Check sheet for the drawn part. Datum: minimum x, y, z corner. Units: mm. A direction names the side the tool comes from. Give positions to 0.01 mm unless a question says otherwise; leave off trailing zeros. Write each loop counter-clockwise with the first axis right and the second up, starting at its lowest first coordinate (ties: lowest second). Pieces come first, ordered by that corner, then holes. Notation, with made-up numbers: (79.25, -36.75) - (121.25, -36.75) arc R28 cw to (121.25, -8.75) - close; hole circle Ø11 at (-3.75, 48.5). An arc over 180 degrees is marked (long way). One line per question, with ' | ' between items. Start each with the question number.
Q1. Section check A-A on x = 37.5. Record the boundary of the cut face in (y, z).
Q2. Thickness scan on L1, parallel to Y at x = 2.5, z = 0.45; L2, parallel to Y at x = 19.5, z = 2.2; L3, parallel to Z at x = 13, y = 2. Record the ranges inside material, lowest first. Write a range as [from, to].
Q3. Section check D-D on y = 24. Record the boundary of the cut face in (x, z), and give its area (3 significant figures).
Q4. Set-up check for the marked faces 1, 2, 3, 4 and 5: record each of +Z, -Z, +X, -X, +Y, -Y from which the full face is reachable in a straight line by a thin tool's end or side.
Q5. Section check B-B on y = 2.5. Record the boundary of the cut face in (x, z), and give its area (3 significant figures).
Q6. Section check C-C on x = 28. Record the boundary of the cut face in (y, z).
Q7. Gauge pin test, flat ends, axial feed: P1, Ø6, axis at x = 16, y = 26, coming from the +Z side; P2, Ø11.5, axis at x = 36, y = 28.5, coming from the +Z side; P3, Ø0.5, axis at y = 24.5, z = 1.5, coming from the -X side; P4, Ø1.8, axis at x = 37.5, y = 2.5, coming from the -Z side. Record the tip position at first contact, or that the pin passes through.
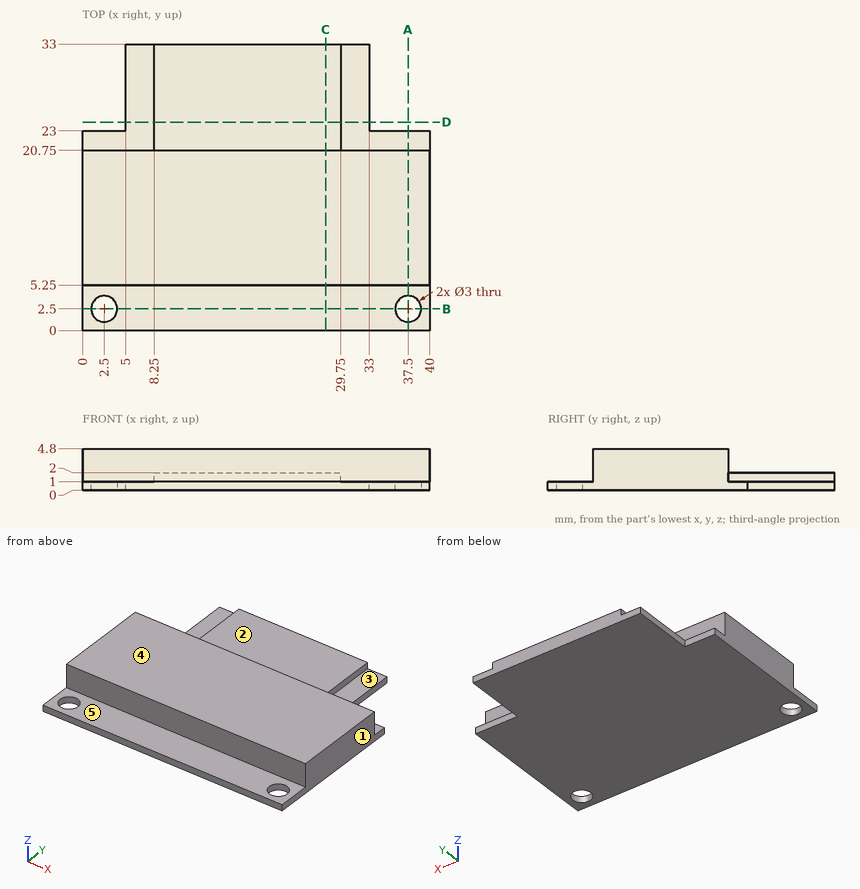
Working result:
1) outline: (0, 0) - (1, 0) - (1, 1) - (0, 1) - close; (4, 0) - (23, 0) - (23, 1) - (20.75, 1) - (20.75, 4.8) - (5.25, 4.8) - (5.25, 1) - (4, 1) - close
2) L1: y = [0, 1], [4, 23] | L2: y = [5.25, 20.75] | L3: z = [0, 1]
3) outline: (5, 0) - (33, 0) - (33, 1) - (29.75, 1) - (29.75, 2) - (8.25, 2) - (8.25, 1) - (5, 1) - close | area: 49.5 mm2
4) face 1: +Z, -Z, +X, +Y, -Y | face 2: +Z, +X, -X, +Y | face 3: +Z, +X, +Y | face 4: +Z, +X, -X, +Y, -Y | face 5: +Z, +X, -X, -Y
5) outline: (0, 0) - (1, 0) - (1, 1) - (0, 1) - close; (4, 0) - (36, 0) - (36, 1) - (4, 1) - close; (39, 0) - (40, 0) - (40, 1) - (39, 1) - close | area: 34.0 mm2
6) outline: (0, 0) - (33, 0) - (33, 2) - (20.75, 2) - (20.75, 4.8) - (5.25, 4.8) - (5.25, 1) - (0, 1) - close
7) P1: stops at z = 2 | P2: stops at z = 1 | P3: stops at x = 8.25 | P4: passes through
